```python
from build123d import *

# Parameters (mm, degrees)
SKETCH1_R               = 50
BOSS_EXTRUDE1_DEPTH     = 45
SKETCH2_R               = 2.5
CUT_EXTRUDE1_DEPTH      = 41
SKETCH3_W               = 8.5
SKETCH3_H               = 20.5
SKETCH3_R               = 1.5
CUT_EXTRUDE2_DEPTH      = 14
SKETCH3_3_R             = 1.5
CUT_EXTRUDE3_DEPTH      = 19
SKETCH3_4_W             = 67
SKETCH3_4_H             = 30.5
SKETCH3_4_W_2           = 8.5
SKETCH3_4_H_2           = 20.5
SKETCH3_4_R             = 1.5
SKETCH3_4_W_3           = 40
CUT_EXTRUDE4_DEPTH      = 87
CUT_EXTRUDE5_DEPTH      = 198.034718556
CUT_EXTRUDE5_DEPTH_BACK = 40
CUT_EXTRUDE6_DEPTH      = 146


with BuildPart() as part:
    # Sketch1 → Boss-Extrude1 (new body)
    with BuildSketch(Plane(origin=(0, 0, 0), x_dir=(1, 0, 0), z_dir=(0, 1, 0))):
        Circle(SKETCH1_R)
        with BuildLine():
            Line((150, 50), (0, 50))
            ThreePointArc((0, 50), (35.355339059, 35.355339059), (50, 0))
            ThreePointArc((50, 0), (35.355339059, -35.355339059), (0, -50))
            Line((0, -50), (150, -50))
            Line((150, -50), (185.196329112, -14.803670888))
            Line((185.196329112, -14.803670888), (185.196329112, 14.803670888))
            Line((185.196329112, 14.803670888), (150, 50))
        make_face()
    extrude(amount=-BOSS_EXTRUDE1_DEPTH)

    # Sketch2 → Cut-Extrude1 (cut)
    # profile 1 of 3: a face of its own
    with BuildSketch(Plane(origin=(0, 0, 0), x_dir=(1, 0, 0), z_dir=(0, 1, 0))):
        with BuildLine():
            Line((4.5, -10.25), (22.214337625, -10.25))
            ThreePointArc((22.214337625, -10.25), (18.5, 0), (22.214337625, 10.25))
            Line((22.214337625, 10.25), (4.5, 10.25))
            Line((4.5, 10.25), (4.5, -10.25))
        make_face()
    # profile 2 of 3: a face of its own
    with BuildSketch(Plane(origin=(0, 0, 0), x_dir=(1, 0, 0), z_dir=(0, 1, 0))):
        with BuildLine():
            Line((22.214337625, -10.25), (44.5, -10.25))
            Line((44.5, -10.25), (44.5, 10.25))
            Line((44.5, 10.25), (22.214337625, 10.25))
            ThreePointArc((22.214337625, 10.25), (18.5, 0), (22.214337625, -10.25))
        make_face()
        with Locations((34.5, 0)):
            Circle(SKETCH2_R, mode=Mode.SUBTRACT)
    # profile 3 of 3: a face of its own
    with BuildSketch(Plane(origin=(0, 0, 0), x_dir=(1, 0, 0), z_dir=(0, 1, 0))):
        with Locations((34.5, 0)):
            Circle(SKETCH2_R)
    extrude(amount=-CUT_EXTRUDE1_DEPTH, mode=Mode.SUBTRACT)

    # Sketch3 → Cut-Extrude2 (cut)
    # profile 1 of 2: a face of its own
    with BuildSketch(Plane(origin=(0, 0, 0), x_dir=(1, 0, 0), z_dir=(0, 1, 0))):
        with Locations((0.25, 0)):
            Rectangle(SKETCH3_W, SKETCH3_H)
        with Locations(Location((0.5, -5, 0), (0, 0, 270))):
            Circle(SKETCH3_R, mode=Mode.SUBTRACT)
        with Locations(Location((0.5, 5, 0), (0, 0, 270))):
            Circle(SKETCH3_R, mode=Mode.SUBTRACT)
    # profile 2 of 2: a face of its own
    with BuildSketch(Plane(origin=(0, 0, 0), x_dir=(1, 0, 0), z_dir=(0, 1, 0))):
        with Locations((48.75, 0)):
            Rectangle(SKETCH3_W, SKETCH3_H)
        with Locations(Location((48.5, -5, 0), (0, 0, 270))):
            Circle(SKETCH3_R, mode=Mode.SUBTRACT)
        with Locations(Location((48.5, 5, 0), (0, 0, 270))):
            Circle(SKETCH3_R, mode=Mode.SUBTRACT)
    extrude(amount=-CUT_EXTRUDE2_DEPTH, mode=Mode.SUBTRACT)

    # Sketch3_3 → Cut-Extrude3 (cut)
    with BuildSketch(Plane(origin=(0, 0, 0), x_dir=(1, 0, 0), z_dir=(0, 1, 0))):
        with Locations(Location((0.5, 5, 0), (0, 0, 270))):
            Circle(SKETCH3_3_R)
        with Locations(Location((0.5, -5, 0), (0, 0, 270))):
            Circle(SKETCH3_3_R)
        with Locations(Location((48.5, 5, 0), (0, 0, 270))):
            Circle(SKETCH3_3_R)
        with Locations(Location((48.5, -5, 0), (0, 0, 270))):
            Circle(SKETCH3_3_R)
    extrude(amount=-CUT_EXTRUDE3_DEPTH, mode=Mode.SUBTRACT)

    # Sketch3_4 → Cut-Extrude4 (cut)
    # profile 1 of 10: a face of its own
    with BuildSketch(Plane(origin=(0, 0, 0), x_dir=(1, 0, 0), z_dir=(0, 1, 0))):
        with BuildLine():
            Line((0, 50), (58, 15.25))
            Line((58, 15.25), (-9, 15.25))
            Line((-9, 15.25), (-9, -15.25))
            Line((-9, -15.25), (58, -15.25))
            Line((58, -15.25), (0, -50))
            ThreePointArc((0, -50), (-50, 0), (0, 50))
        make_face()
        with BuildLine():
            ThreePointArc((-33.081762137, 18.240700348), (-31.348197127, 11.810741084), (-24.918237863, 13.544306095))
            ThreePointArc((-24.918237863, 13.544306095), (-14.201955248, 24.13017398), (0.428262315, 27.715706859))
            ThreePointArc((0.428262315, 27.715706859), (5.272422948, 32.285579018), (0.702550789, 37.129739651))
            ThreePointArc((0.702550789, 37.129739651), (-18.798044752, 32.350588133), (-33.081762137, 18.240700348))
        make_face(mode=Mode.SUBTRACT)
    # profile 2 of 10: a face of its own
    with BuildSketch(Plane(origin=(0, 0, 0), x_dir=(1, 0, 0), z_dir=(0, 1, 0))):
        with Locations((24.5, 0)):
            Rectangle(SKETCH3_4_W, SKETCH3_4_H)
        Polygon((53, -10.25), (44.5, -10.25), (4.5, -10.25), (-4, -10.25), (-4, 10.25), (4.5, 10.25), (44.5, 10.25), (53, 10.25), align=None, mode=Mode.SUBTRACT)
    # profile 3 of 10: a face of its own
    with BuildSketch(Plane(origin=(0, 0, 0), x_dir=(1, 0, 0), z_dir=(0, 1, 0))):
        with Locations((48.75, 0)):
            Rectangle(SKETCH3_4_W_2, SKETCH3_4_H_2)
        with Locations((48.5, -5)):
            Circle(SKETCH3_4_R, mode=Mode.SUBTRACT)
        with Locations((48.5, 5)):
            Circle(SKETCH3_4_R, mode=Mode.SUBTRACT)
    # profile 4 of 10: a face of its own
    with BuildSketch(Plane(origin=(0, 0, 0), x_dir=(1, 0, 0), z_dir=(0, 1, 0))):
        with Locations((24.5, 0)):
            Rectangle(SKETCH3_4_W_3, SKETCH3_4_H_2)
    # profile 5 of 10: a face of its own
    with BuildSketch(Plane(origin=(0, 0, 0), x_dir=(1, 0, 0), z_dir=(0, 1, 0))):
        with Locations((0.25, 0)):
            Rectangle(SKETCH3_4_W_2, SKETCH3_4_H_2)
        with Locations((0.5, -5)):
            Circle(SKETCH3_4_R, mode=Mode.SUBTRACT)
        with Locations((0.5, 5)):
            Circle(SKETCH3_4_R, mode=Mode.SUBTRACT)
    # profile 6 of 10: a face of its own
    with BuildSketch(Plane(origin=(0, 0, 0), x_dir=(1, 0, 0), z_dir=(0, 1, 0))):
        with Locations((0.5, 5)):
            Circle(SKETCH3_4_R)
    # profile 7 of 10: a face of its own
    with BuildSketch(Plane(origin=(0, 0, 0), x_dir=(1, 0, 0), z_dir=(0, 1, 0))):
        with Locations((0.5, -5)):
            Circle(SKETCH3_4_R)
    # profile 8 of 10: a face of its own
    with BuildSketch(Plane(origin=(0, 0, 0), x_dir=(1, 0, 0), z_dir=(0, 1, 0))):
        with BuildLine():
            ThreePointArc((0.702550789, 37.129739651), (-18.798044752, 32.350588133), (-33.081762137, 18.240700348))
            ThreePointArc((-33.081762137, 18.240700348), (-31.348197127, 11.810741084), (-24.918237863, 13.544306095))
            ThreePointArc((-24.918237863, 13.544306095), (-14.201955248, 24.13017398), (0.428262315, 27.715706859))
            ThreePointArc((0.428262315, 27.715706859), (5.272422948, 32.285579018), (0.702550789, 37.129739651))
        make_face()
    # profile 9 of 10: a face of its own
    with BuildSketch(Plane(origin=(0, 0, 0), x_dir=(1, 0, 0), z_dir=(0, 1, 0))):
        with Locations((48.5, 5)):
            Circle(SKETCH3_4_R)
    # profile 10 of 10: a face of its own
    with BuildSketch(Plane(origin=(0, 0, 0), x_dir=(1, 0, 0), z_dir=(0, 1, 0))):
        with Locations((48.5, -5)):
            Circle(SKETCH3_4_R)
    extrude(amount=-CUT_EXTRUDE4_DEPTH, mode=Mode.SUBTRACT)

    # Sketch5 → Cut-Extrude5 (cut, two sides: drawn at the far end of the back side and taken through both)
    with BuildSketch(Plane.XZ.offset(45).offset(-CUT_EXTRUDE5_DEPTH_BACK)):
        Polygon((36.14772109, 40), (16.690647482, 40), (58, 15.25), (58, -15.25), (16.690647482, -40), (36.14772109, -40), (145.857864376, -40), (175.196329112, -10.661535265), (175.196329112, 10.661535265), (145.857864376, 40), align=None)
    extrude(amount=CUT_EXTRUDE5_DEPTH + CUT_EXTRUDE5_DEPTH_BACK, mode=Mode.SUBTRACT)

    # Sketch6 → Cut-Extrude6 (cut)
    with BuildSketch(Plane.ZY):
        Polygon((43, -45), (47, -45), (48, -43), (42, -43), align=None)
    cut_extrude6 = extrude(amount=-CUT_EXTRUDE6_DEPTH, mode=Mode.SUBTRACT)

    # Mirror1: Cut-Extrude6 across plane
    add(cut_extrude6.mirror(Plane.XY), mode=Mode.SUBTRACT)


solid = part.part
```
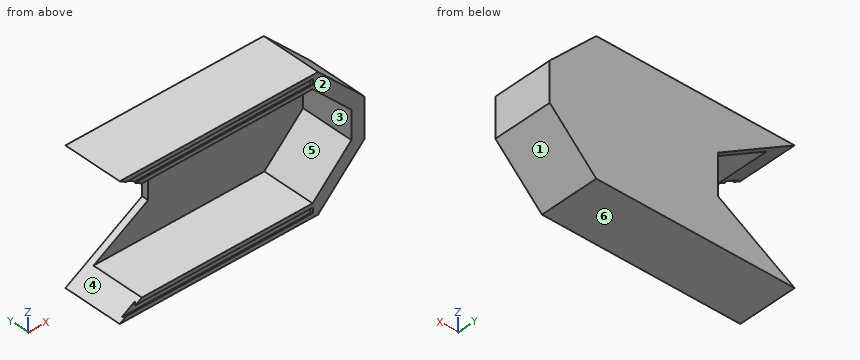
Geometry check sheet. Reference: the model listing, model coordinates, mm. Face numbers are marked on the shaded views. A direction names the side the tool comes from. Coordinates: 2 decimals unless noted, no trailing zeros. Order: outer loops, then holes, each group sorted by start corner. A loop starts at its lowest first (then second) coordinate and runs counter-clockwise, first axis right, second up.
Q1. Thickness scan on probe 1 along Z at (x, y) = (35, -10); probe 2 along X at (y, z) = (-28.5, -4.5); probe 3 along Z at (x, y) = (45, -2). Record the ranges inside material, lowest first.
Reply:
probe 1: z = -50 to -40, 40 to 50
probe 2: x = 175.2 to 185.2
probe 3: z = -50 to -23.04, 23.04 to 50
Q2. Sectioned sample at D-D on x = 165. Record the cut outline in (y, z), and give its area (3 significant figures).
Reply:
outline: (-45, -35) - (0, -35) - (0, 35) - (-45, 35) - (-45, 20.86) - (-5, 20.86) - (-5, -20.86) - (-45, -20.86) - close
area: 1,480 mm2
Q3. Sectioned sample at A-A on x = 46. Record the cut outline in (y, z).
Reply:
outline: (-45, -50) - (0, -50) - (0, -22.44) - (-5, -22.44) - (-5, -40) - (-45, -40) - (-45, -43) - (-43, -42) - (-43, -48) - (-45, -47) - close; (-45, 40) - (-5, 40) - (-5, 22.44) - (0, 22.44) - (0, 50) - (-45, 50) - (-45, 47) - (-43, 48) - (-43, 42) - (-45, 43) - close
Q4. Draft check along Z on the marked faces 1, 2 and 3. Enter one of: released by +Z, released by -Z, zero draft, split by the parting line, or undercut.
Reply:
face 1: released by -Z
face 2: zero draft
face 3: undercut
Q5. Sectioned sample at C-C on z = -4.5. Record the cut outline in (x, y), and give its area (3 significant figures).
Reply:
outline: (58, -5) - (175.2, -5) - (175.2, -45) - (185.2, -45) - (185.2, 0) - (58, 0) - close
area: 1,040 mm2
Q6. Sectioned sample at B-B on y = -24.5. Record the cut outline in (x, z), and give its area (3 significant figures).
Reply:
outline: (0, -50) - (150, -50) - (185.2, -14.8) - (185.2, 14.8) - (150, 50) - (0, 50) - (16.69, 40) - (145.86, 40) - (175.2, 10.66) - (175.2, -10.66) - (145.86, -40) - (16.69, -40) - close
area: 3,960 mm2
Q7. Tool access check on the marked faces 4, 5 and 6. Record the directions out of +Z, -Z, +X, -X, +Y, -Y that give a thin tool (end or side, any length) a straight path to the whole face; none if there is none.
Reply:
face 4: -X, +Y, -Y
face 5: -X, -Y
face 6: -Z, +X, -X, +Y, -Y
Q8. Depth check by flat-ended pin: pin 1 Ø1 at (y, z) = (-14.5, 18) entering from +X; pin 2 Ø1 at (y, z) = (-44.5, 44.5) entering from -X; pin 3 Ø5 at (x, z) = (112, -28.5) entering from -Y. Enter the tip coordinate at first touch or a pass-through.
Reply:
pin 1: stops at x = 182.5
pin 2: stops at x = 146
pin 3: stops at y = -5
